Autodesk Inventor part; units mm, degrees
ref_plane "YZ Plane" through (0, 0, 0) normal (1, 0, 0) x (0, 1, 0)
ref_plane "XZ Plane" through (0, 0, 0) normal (0, 1, 0) x (-1, 0, 0)
ref_plane "XY Plane" through (0, 0, 0) normal (0, 0, 1) x (1, 0, 0)
ref_plane "Work Plane2" through (0, 0, 0) normal (0, 0, 1) x (1, 0, 0)
sketch "Sketch1" plane through (0, 0, 0) normal (0, 0, 1) x (1, 0, 0)
  line L0 (29.5603, 0.0547) -> (16.8603, 0.0547)
  line L1 (16.8603, 0.0547) -> (16.8603, 40.6947)
  line L2 (16.8603, 40.6947) -> (29.5603, 40.6947)
  line L3 (29.5603, 40.6947) -> (29.5603, 0.0547)
  point P0 (0, 0)
  dimension "d0" = 12.7
  dimension "d1" = 40.64
extrude "Extrusion1" add sketch "Sketch1" along normal blind 12.7
sketch "Sketch2" plane through (16.8603, 40.6947, 0) normal (0, 1, 0) x (1, 0, 0)
  circle A0 centre (6.35, -31.115) radius 18.415
  line L0 (12.7, -12.7) -> (0, -12.7)
  line L1 (0, 0) -> (0, -12.7)
  circle A1 centre (6.35, -31.115) radius 22.86
  point P0 (-16.8603, 0)
  point P1 (6.35, -12.7)
  dimension "d4" = 36.83
  dimension "d6" = 6.35
  dimension "d7" = 45.72
extrude "Extrusion2" add sketch "Sketch2" against normal blind 40.64
sketch "Sketch3" plane through (16.8603, 40.6947, 0) normal (0, 1, 0) x (1, 0, 0)
  circle A0 centre (6.35, -31.115) radius 18.415
  circle A1 centre (6.35, -31.115) radius 18.415
  circle A2 centre (21.844, -31.115) radius 1.9939
  circle A3 centre (-9.144, -31.115) radius 1.9939
  circle A4 centre (6.35, -38.1254) radius 6.096
  point P0 (-16.8603, 0)
  point P1 (2.6162, -31.115)
  dimension "d10" = 36.83
  dimension "d21" = 3.9878
  dimension "d22" = 3.9878
  dimension "d23" = 30.988
  dimension "d27" = 12.192
  dimension "d28" = 7.0104
extrude "Extrusion3" add sketch "Sketch3" against normal blind 4.318
sketch "Sketch6" plane through (0, 0, 0) normal (0, 0, -1) x (-1, 0, 0)
  line L0 (-16.8603, 0.0547) -> (-2.8903, 0.0547)
  line L1 (-2.8903, 0.0547) -> (-2.8903, 40.6947)
  line L2 (-2.8903, 40.6947) -> (-16.8603, 40.6947)
  line L3 (-16.8603, 40.6947) -> (-16.8603, 0.0547)
  point P0 (0, 0)
  dimension "d36" = 13.97
  dimension "d37" = 40.64
extrude "Extrusion4" add sketch "Sketch6" against normal up to next
sketch "Sketch7" plane through (0, 0, 0) normal (0, 0, -1) x (-1, 0, 0)
  line L0 (-29.5603, 40.6947) -> (-29.5603, 0.0547)
  line L1 (-46.0703, 40.6947) -> (-0.3503, 40.6947)
  line L2 (-29.5603, 0.0547) -> (-43.5303, 0.0547)
  line L3 (-43.5303, 0.0547) -> (-43.5303, 40.6947)
  line L4 (-43.5303, 40.6947) -> (-29.5603, 40.6947)
  line L5 (-29.5603, 40.6947) -> (-29.5603, 0.0547)
  point P0 (0, 0)
  point P1 (-2.8903, 40.6947)
  dimension "d40" = 13.97
extrude "Extrusion5" add sketch "Sketch7" against normal up to next
properties part number "Suspension Bracket Mount"
The listing builds one solid part. Answer for the finished solid, in the listing's coordinates (mm). A direction names the side the tool comes from. Give positions to 0.01 mm unless a question says otherwise; leave off trailing zeros. Order: outer loops, then holes, each group sorted by start corner. A loop starts at its lowest first (then second) coordinate and runs counter-clockwise, first axis right, second up. Notation, with made-up numbers: (7, 33.5) - (23, 33.5) arc R32 ccw to (23, 59.5) - close; hole circle Ø1 at (-16, -10). An arc over 180 degrees is marked (long way). One line per item, written item: value. Start each with the question number.
1) Given pin 1 Ø2.5 at (x, z) = (7.72, 31.12) entering from -Y; pin 2 Ø4 at (y, z) = (13, 46) entering from +X; pin 3 Ø10.5 at (y, z) = (20, 15.5) entering from +X; pin 4 Ø4 at (y, z) = (23.5, 35.5) entering from -X, each flat-ended and moving along its own axis, determine where each tip first touches the part or whether it passes through.
2) Find the intervals of material crossed by L1, parallel to Z at x = 22.5, y = 24; L2, parallel to Y at x = 18.5, z = 25; L3, parallel to X at y = 3, z = 14, in increasing order.
3) The mould has two halves that part along X. Classify faces 1 (the face through (2.89, 20, 10)), 2 (the face through (40.775, 18.47, 25.584)), 3 (the face through (23, 21, 0)): released by +X, released by -X, zero draft, split by the parting line, or undercut.
4) A cutting plane is placed at D-D on z = 17.5. Give the vertices of the cut face in (x, y), then the cut area to 3 significant figures.
5) A cutting plane is placed at A-A on x = 38. Give the vertices of the cut face in (y, z).
6) A cutting plane is placed at C-C on x = 30.5. Give the vertices of the cut face in (y, z), then the cut area to 3 significant figures.
7) A cutting plane is placed at B-B on z = 43.5. Give the vertices of the cut face in (x, y), then the cut area to 3 significant figures.
8) A tool of negligible diameter and unlimited length cuts with its end or side. For faces 4 (the face through (8.64, 38.57, 32.88)), 5 (the face through (23, 36.377, 31)), 6 (the face through (43.53, 20, 10)), from which of +Z, -Z, +X, -X, +Y, -Y can it reach the whole face along a straight path? Write none if from no direction.
Answer sheet:
1. pin 1: passes through
1. pin 2: stops at x = 42.09
1. pin 3: stops at x = 43.59
1. pin 4: stops at x = 0.48
2. L1: z = 0 to 12.71, 49.52 to 53.96
2. L2: y = 36.38 to 40.69
2. L3: x = 2.89 to 16.41, 30.01 to 43.53
3. face 1: released by -X
3. face 2: undercut
3. face 3: zero draft
4. outline: (2.89, 0.05) - (10.81, 0.05) - (10.81, 36.38) - (35.61, 36.38) - (35.61, 0.05) - (43.53, 0.05) - (43.53, 40.69) - (2.89, 40.69) - close
4. area: 751 mm2
5. outline: (0.05, 0) - (40.69, 0) - (40.69, 29.25) - (36.38, 29.25) - (36.38, 20.14) - (0.05, 20.14) - close; (0.05, 42.09) - (36.38, 42.09) - (36.38, 32.98) - (40.69, 32.98) - (40.69, 48.55) - (0.05, 48.55) - close
6. outline: (0.05, 0) - (40.69, 0) - (40.69, 52.78) - (0.05, 52.78) - (0.05, 48.03) - (36.38, 48.03) - (36.38, 14.2) - (0.05, 14.2) - close
6. area: 917 mm2
7. outline: (4, 0.05) - (9.58, 0.05) - (9.58, 36.38) - (20.33, 36.38) - (20.33, 40.69) - (4, 40.69) - close; (26.09, 36.38) - (36.84, 36.38) - (36.84, 0.05) - (42.42, 0.05) - (42.42, 40.69) - (26.09, 40.69) - close
7. area: 547 mm2
8. face 4: +Y, -Y
8. face 5: -Y
8. face 6: -Z, +X, +Y, -Y
